Autodesk Inventor part; units mm, degrees
ref_plane "YZ Plane" through (0, 0, 0) normal (1, 0, 0) x (0, 1, 0)
ref_plane "XZ Plane" through (0, 0, 0) normal (0, 1, 0) x (-1, 0, 0)
ref_plane "XY Plane" through (0, 0, 0) normal (0, 0, 1) x (1, 0, 0)
sketch "Sketch1" plane through (0, 0, 0) normal (0, 0, 1) x (1, 0, 0)
  circle A0 centre (0, 0) radius 30.16
  circle A1 centre (0, 0) radius 17.5
  dimension "d0" = 60.32
  dimension "d1" = 35
extrude "Extrusion1" add sketch "Sketch1" along normal blind 24.8
sketch "Sketch2" plane through (0, 0, 24.8) normal (0, 0, 1) x (1, 0, 0)
  circle A0 centre (0, 0) radius 25
  dimension "d4" = 50
extrude "Extrusion2" add sketch "Sketch2" along normal blind 5
sketch "Sketch3" plane through (0, 0, 29.8) normal (0, 0, 1) x (1, 0, 0)
  circle A0 centre (0, 0) radius 17.5
  dimension "d7" = 35
extrude "Extrusion3" cut sketch "Sketch3" against normal blind 71.75
fillet "Fillet1" radius 0.5 1 edges at (-30.16, 0, 24.8)
fillet "Fillet2" radius 0.5 3 edges at (-30.16, 0, 0) (-25, 0, 29.8) (-17.5, 0, 0)
properties part number "coração do homem de ferro"
Geometry: final body of the model. Coordinates: model frame, mm. A direction names the side the tool comes from. Round coordinates to 2 decimals unless told otherwise and drop trailing zeros. Order: outer loops, then holes, each group sorted by start corner. A loop starts at its lowest first (then second) coordinate and runs counter-clockwise, first axis right, second up. Notation, with made-up numbers: M 4,29 L 16,29 A14 cw 16,47 Z; hole C 36,71.25 d5. An arc over 180 degrees is marked long. One line per item, written item: value.
(1) Line query: probe 1 along Y at (x, z) = (0, 15); probe 2 along Z at (x, y) = (-8.5, 27.5); probe 3 along Y at (x, z) = (-5, 12.5). Output: solid intervals per line, ascending. Write a range as [from, to].
Result sheet:
probe 1: [-30.16, -17.5], [17.5, 30.16]
probe 2: [0, 24.8]
probe 3: [-29.74, -16.77], [16.77, 29.74]
(2) Reachability of faces 4 (the flat face through (-16, -20, 24.8)), 5 (the cylindrical face through (13.917, 26.757, 12.233)) from +Z, -Z, +X, -X, +Y, -Y: full face, straight path, thin tool, end or side. Return the list, or none.
Result sheet:
face 4: +Z
face 5: +Z, -Z
(3) Pull-direction query (X, two-part tool) for faces 1 (the flat face through (-17, 6, 29.8)), 2 (the cylindrical face through (23.846, -7.509, 27.018)), 3 (the cylindrical face through (-13.887, 10.648, 14.945)); classes: pulls with the +X half, pulls with the -X half, needs draft (parallel to the pull), parting line crosses it, or undercut.
Result sheet:
face 1: needs draft
face 2: parting line crosses it
face 3: undercut
(4) Cut plane A-A (y = 0). Return the cut outline in (x, z).
Result sheet:
outline: M -30.16,0.5 A0.5 ccw -29.66,0 L -18,0 A0.5 ccw -17.5,0.5 L -17.5,29.8 L -24.5,29.8 A0.5 ccw -25,29.3 L -25,24.8 L -29.66,24.8 A0.5 ccw -30.16,24.3 Z; M 17.5,0.5 A0.5 ccw 18,0 L 29.66,0 A0.5 ccw 30.16,0.5 L 30.16,24.3 A0.5 ccw 29.66,24.8 L 25,24.8 L 25,29.3 A0.5 ccw 24.5,29.8 L 17.5,29.8 Z
(5) Cut plane C-C (z = 27.75). Return the cut outline in (x, y).
Result sheet:
outline: C 0,0 d50; hole C 0,0 d35
(6) Pin query (flat end, axial travel): P1, Ø8, axis at x = -22.5, y = -22.5, coming from the +Z side; P2, Ø3, axis at x = -19.5, z = 13, coming from the -Y side; P3, Ø3, axis at y = -21, z = 6, coming from the +X side. Return the tip coordinate at first contact, or that it passes through.
Result sheet:
P1: z = 24.8
P2: y = -24.2
P3: x = 23.01
(7) Cut plane D-D (z = 13.5). Return the cut outline in (x, y).
Result sheet:
outline: C 0,0 d60.32; hole C 0,0 d35
